Here's how the part is built. I have some questions about the finished solid (model axes, mm). A direction names the side the tool comes from. Round coordinates to 2 decimals unless told otherwise and drop trailing zeros. Order: outer loops, then holes, each group sorted by start corner. A loop starts at its lowest first (then second) coordinate and runs counter-clockwise, first axis right, second up. Notation, with made-up numbers: M 54,-23.5 L 81,-23.5 A22 cw 81,12.5 Z; hole C -23.5,88 d4. An arc over 180 degrees is marked long. Write item = value, one per line. Start each with the question number.
Item 1: I want a section at A-A, the plane z = 9. List the corners of the cut face in (x, y) for me.
Item 2: We'd pull the mould along Y, two halves only. Please class faces 6 (the face through (40, 223, 0)), 7 (the face through (0, 10, 3)), 8 (the face through (-1, 453, 4)): pulls with the +Y half, pulls with the -Y half, needs draft (parallel to the pull), parting line crosses it, or undercut.
Item 3: Please list where these lines run through material, in increasing order: L1, parallel to Y at x = -18, z = 4.1; L2, parallel to Y at x = -1, z = 1.5; L3, parallel to X at y = 416.5, z = 1.5.
Item 4: For faces 1 (the face through (-54, 223, 0.4)), 2 (the face through (47, 223, 5.5)), 3 (the face through (0, 223, 0.4)), 4 (the face through (54, 223, 0.4)), 5 (the face through (0, 45, 3)), which set-ups out of +Z, -Z, +X, -X, +Y, -Y let a thin tool reach every point of the face, with its end or its side?
Item 5: I'm going to push flat-ended pins straight in: P1, Ø6, axis at y = 101.5, z = 5.5, coming from the +X side; P2, Ø2.5, axis at y = 27.5, z = 4, coming from the -X side; P3, Ø4, axis at y = 30, z = 3.5, coming from the +X side. Where does each tip first touch, or does it pass through?
```python
from build123d import *

# Parameters (mm, degrees)
BOSS_EXTRUDE1_DEPTH      = 253
BOSS_EXTRUDE1_DEPTH_BACK = 200
SKETCH2_R                = 2.75
CUT_EXTRUDE1_DEPTH       = 458.853688421
SKETCH3_R                = 2.1
CUT_EXTRUDE2_DEPTH       = 458.853688421
CUT_EXTRUDE3_DEPTH       = 458.841632009


# Read off the part's stored shape, not the designer's step: Imported1
with BuildPart() as part:
    # Sketch1 → Boss-Extrude1 (new, two sides: drawn at the far end of the back side and taken through both)
    with BuildSketch(Plane(origin=(0, 200, 0), x_dir=(1, 0, 0), z_dir=(0, 1, 0)).offset(-BOSS_EXTRUDE1_DEPTH_BACK)):
        with BuildLine():
            Line((0, -5.21132487), (0.5, -5.5))
            Line((0.5, -5.5), (39.5, -5.5))
            Line((39.5, -5.5), (40, -5.21132487))
            Line((40, -5.21132487), (40.5, -5.5))
            Line((40.5, -5.5), (54, -5.5))
            Line((54, -5.5), (55.431521652, -6.326489411))
            ThreePointArc((55.431521652, -6.326489411), (55.569235651, -6.501322592), (55.548605331, -6.722921727))
            ThreePointArc((55.548605331, -6.722921727), (62.487270984, -13.337451224), (60.283018873, -4.0080164))
            ThreePointArc((60.283018873, -4.0080164), (60.081946867, -3.914538227), (60, -3.708497377))
            Line((60, -3.708497377), (60, -0.9))
            Line((60, -0.9), (59.5, -0.4))
            Line((59.5, -0.4), (48.4, -0.4))
            Line((48.4, -0.4), (48, 0))
            Line((48, 0), (32, 0))
            Line((32, 0), (31.6, -0.4))
            Line((31.6, -0.4), (-31.6, -0.4))
            Line((-31.6, -0.4), (-32, 0))
            Line((-32, 0), (-48, 0))
            Line((-48, 0), (-48.4, -0.4))
            Line((-48.4, -0.4), (-59.5, -0.4))
            Line((-59.5, -0.4), (-60, -0.9))
            Line((-60, -0.9), (-60, -3.708497387))
            ThreePointArc((-60, -3.708497387), (-60.081946862, -3.914538232), (-60.283018865, -4.0080164))
            ThreePointArc((-60.283018865, -4.0080164), (-62.487270987, -13.337451222), (-55.548605331, -6.722921727))
            ThreePointArc((-55.548605331, -6.722921727), (-55.569235651, -6.501322592), (-55.431521652, -6.326489411))
            Line((-55.431521652, -6.326489411), (-54, -5.5))
            Line((-54, -5.5), (-40.5, -5.5))
            Line((-40.5, -5.5), (-40, -5.21132487))
            Line((-40, -5.21132487), (-39.5, -5.5))
            Line((-39.5, -5.5), (-0.5, -5.5))
            Line((-0.5, -5.5), (0, -5.21132487))
        make_face()
    extrude(amount=BOSS_EXTRUDE1_DEPTH + BOSS_EXTRUDE1_DEPTH_BACK)

    # Sketch2 → Cut-Extrude1 (cut, through all)
    with BuildSketch(Plane(origin=(0, 0, 0), x_dir=(-1, 0, 0), z_dir=(0, 0, -1))):
        with Locations((-18, 415.5)):
            Circle(SKETCH2_R)
        with Locations((18, 415.5)):
            Circle(SKETCH2_R)
        with Locations((-18, 37.5)):
            Circle(SKETCH2_R)
        with Locations((18, 37.5)):
            Circle(SKETCH2_R)
        with Locations((-41, 447.5)):
            Circle(SKETCH2_R)
        with Locations((-18, 447.5)):
            Circle(SKETCH2_R)
        with Locations((18, 447.5)):
            Circle(SKETCH2_R)
        with Locations((41, 447.5)):
            Circle(SKETCH2_R)
        with Locations(Location((-41, 5.5, 0), (0, 0, 303.055731151))):
            Circle(SKETCH2_R)
        with Locations((-18, 5.5)):
            Circle(SKETCH2_R)
        with Locations((18, 5.5)):
            Circle(SKETCH2_R)
        with Locations(Location((41, 5.5, 0), (0, 0, 100.475681696))):
            Circle(SKETCH2_R)
    extrude(amount=-CUT_EXTRUDE1_DEPTH, mode=Mode.SUBTRACT)

    # Sketch3 → Cut-Extrude2 (cut, through all)
    with BuildSketch(Plane(origin=(0, 0, 0), x_dir=(-1, 0, 0), z_dir=(0, 0, -1))):
        with Locations((-42.3, 413.77)):
            Circle(SKETCH3_R)
        with Locations((42.7, 413.77)):
            Circle(SKETCH3_R)
        with Locations(Location((-42.3, 39.23, 0), (0, 0, 31.002719134))):
            Circle(SKETCH3_R)
        with Locations((42.7, 39.23)):
            Circle(SKETCH3_R)
    extrude(amount=-CUT_EXTRUDE2_DEPTH, mode=Mode.SUBTRACT)

    # Sketch4 → Cut-Extrude3 (cut, through all)
    with BuildSketch(Plane(origin=(0, 0, 0.4), x_dir=(-1, 0, 0), z_dir=(0, 0, -1))):
        with BuildLine():
            Line((10, 35), (10, 20))
            ThreePointArc((10, 20), (0, 10), (-10, 20))
            Line((-10, 20), (-10, 35))
            ThreePointArc((-10, 35), (0, 45), (10, 35))
        make_face()
    extrude(amount=-CUT_EXTRUDE3_DEPTH, mode=Mode.SUBTRACT)


solid = part.part
```
Filled in:
q1.outline = M -65,0 L -55,0 L -55,453 L -65,453 Z; M 55,0 L 65,0 L 65,453 L 55,453 Z
q2.face_6 = needs draft
q2.face_7 = undercut
q2.face_8 = pulls with the +Y half
q3.L1 = 0 to 2.75, 8.25 to 34.75, 40.25 to 412.75, 418.25 to 444.75, 450.25 to 453
q3.L2 = 0 to 10.05, 44.95 to 453
q3.L3 = -60 to -20.56, -15.44 to 15.44, 20.56 to 60
q4.face_1 = -Z, -X, +Y, -Y
q4.face_2 = +Z, +Y, -Y
q4.face_3 = -Z, +Y, -Y
q4.face_4 = -Z, +X, +Y, -Y
q4.face_5 = +Z, -Z
q5.P1 = 64.97
q5.P2 = -63.31
q5.P3 = 63.57
